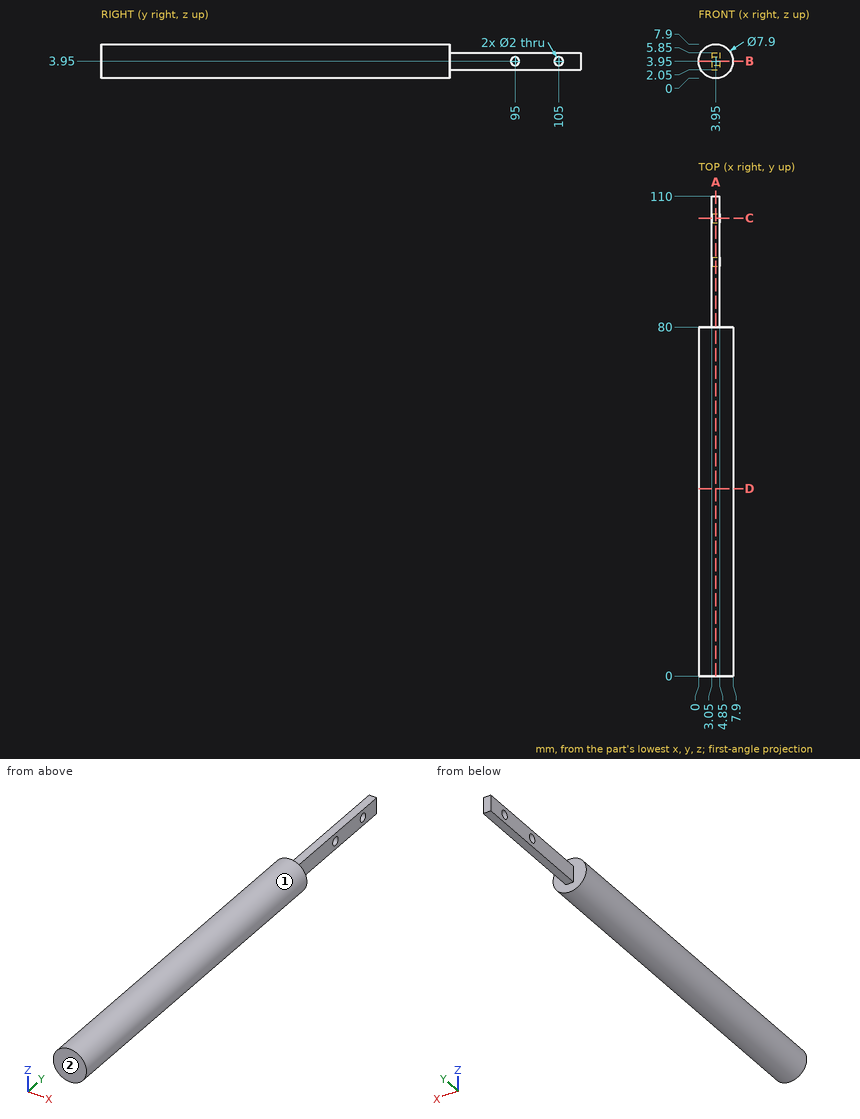
Study the drawing (mm; zero at the part's minimum x, y, z) and answer. Give positions to 0.01 mm unless a question says otherwise; leave off trailing zeros. Write each loop counter-clockwise with the first axis right and the second up, starting at its lowest first coordinate (ties: lowest second). Pieces come first, ordered by that corner, then holes.
Item 1: Section D-D, the plane y = 43 is taken. Write down the section's boundary in (x, z).
Item 2: Find the intervals of material crossed by line 1 along Y through (x, z) = (4.35, 3.95); line 2 along Z through (x, y) = (3.9, 95); line 3 along Y through (x, z) = (7, 5.5), in increasing order.
Item 3: Flat-ended cylindrical pins translate along their axes: P1, Ø1.1, axis at y = 97, z = 4, coming from the +X side; P2, Ø0.5, axis at x = 3.5, y = 98.5, coming from the -Z side; P3, Ø1, axis at x = 5, y = 12.5, coming from the +Z side. Find the tip coordinate at first contact, or state that the pin passes through.
Item 4: Section B-B, the plane z = 3.95 is taken. Write down the section's boundary in (x, y).
Item 5: Determine the mould class of the marked faces 1 and 2 for opening direction X: released by +X, released by -X, zero draft, split by the parting line, or undercut.
Item 6: Section C-C, the plane y = 105 is taken. Write down the section's boundary in (x, z), plus the area to 3 significant figures.
Item 7: Section A-A, the plane x = 3.95 is taken. Write down the section's boundary in (y, z).
Completed:
1. outline: circle Ø7.9 at (3.95, 3.95)
2. line 1: y = 0 to 94, 96 to 104, 106 to 110
2. line 2: z = 2.05 to 2.95, 4.95 to 5.85
2. line 3: y = 0 to 80
3. P1: stops at x = 4.85
3. P2: stops at z = 2.05
3. P3: stops at z = 7.86
4. outline: (0, 0) - (7.9, 0) - (7.9, 80) - (4.85, 80) - (4.85, 94) - (3.05, 94) - (3.05, 80) - (0, 80) - close; (3.05, 96) - (4.85, 96) - (4.85, 104) - (3.05, 104) - close; (3.05, 106) - (4.85, 106) - (4.85, 110) - (3.05, 110) - close
5. face 1: split by the parting line
5. face 2: zero draft
6. outline: (3.05, 2.05) - (4.85, 2.05) - (4.85, 2.95) - (3.05, 2.95) - close; (3.05, 4.95) - (4.85, 4.95) - (4.85, 5.85) - (3.05, 5.85) - close
6. area: 3.24 mm2
7. outline: (0, 0) - (80, 0) - (80, 2.05) - (110, 2.05) - (110, 5.85) - (80, 5.85) - (80, 7.9) - (0, 7.9) - close; hole circle Ø2 at (95, 3.95); hole circle Ø2 at (105, 3.95)
